Could you check a few things on this model? Use its own coordinates, in mm. A direction names the side the tool comes from. Coordinates: 2 decimals unless noted, no trailing zeros. Loops run counter-clockwise (first coordinate to the right, second up) from the corner with the lowest first, then second, coordinate; pieces in that order, holes last. Notation, with made-up numbers: (57, 41.5) -> (104, 41.5) arc R18 ccw to (104, 61.5) -> close; hole circle Ø5 at (63.5, 24). An arc over 180 degrees is marked (long way). One line per question, with ' | ' between items.
from build123d import *

# Parameters (mm, degrees)
SKETCH2_R           = 76.2
BOSS_EXTRUDE1_DEPTH = 50.8
CUT_EXTRUDE1_DEPTH  = 76.2
CUT_EXTRUDE2_DEPTH  = 76.2
SKETCH8_W           = 5.08
SKETCH8_H           = 5.08
CUT_EXTRUDE4_DEPTH  = 50.8
CUT_EXTRUDE5_DEPTH  = 51.8
SKETCH10_R          = 2.159
CUT_EXTRUDE6_DEPTH  = 25.4


with BuildPart() as part:
    # Sketch2 → Boss-Extrude1 (new body)
    with BuildSketch(Plane.XY):
        Circle(SKETCH2_R)
    extrude(amount=BOSS_EXTRUDE1_DEPTH)

    # Sketch4 → Cut-Extrude1 (cut)
    with BuildSketch(Plane.XY.offset(50.8)):
        with BuildLine():
            Line((-75.519629236, 10.16), (75.519629236, 10.16))
            ThreePointArc((75.519629236, 10.16), (0, 76.2), (-75.519629236, 10.16))
        make_face()
    extrude(amount=-CUT_EXTRUDE1_DEPTH, mode=Mode.SUBTRACT)

    # Sketch5 → Cut-Extrude2 (cut)
    with BuildSketch(Plane.XY.offset(50.8)):
        with BuildLine():
            Line((49.396930897, 5.08), (-49.396930897, 5.08))
            Line((-49.396930897, 5.08), (-49.396930897, -51.166371944))
            ThreePointArc((-49.396930897, -51.166371944), (-41.049983197, -58.077132157), (-31.75, -63.639546667))
            Line((-31.75, -63.639546667), (31.75, -63.639546667))
            ThreePointArc((31.75, -63.639546667), (41.049983197, -58.077132157), (49.396930897, -51.166371944))
            Line((49.396930897, -51.166371944), (49.396930897, 5.08))
        make_face()
    extrude(amount=-CUT_EXTRUDE2_DEPTH, mode=Mode.SUBTRACT)

    # Sketch8 → Cut-Extrude4 (cut)
    with BuildSketch(Plane.XY.offset(50.8)):
        with Locations((0, -66.179546667)):
            Rectangle(SKETCH8_W, SKETCH8_H)
    extrude(amount=-CUT_EXTRUDE4_DEPTH, mode=Mode.SUBTRACT)

    # Sketch9 → Cut-Extrude5 (cut, through all)
    with BuildSketch(Plane.XY.offset(50.8)):
        with BuildLine():
            Line((54.476930897, 5.08), (76.030478099, 5.08))
            ThreePointArc((76.030478099, 5.08), (71.480790805, -26.399555791), (54.476930897, -53.279489487))
            Line((54.476930897, -53.279489487), (54.476930897, 5.08))
        make_face()
        with BuildLine():
            Line((-54.476930897, 5.08), (-54.476930897, -53.279489487))
            ThreePointArc((-54.476930897, -53.279489487), (-71.480790805, -26.399555791), (-76.030478099, 5.08))
            Line((-76.030478099, 5.08), (-54.476930897, 5.08))
        make_face()
    extrude(amount=-CUT_EXTRUDE5_DEPTH, mode=Mode.SUBTRACT)

    # Sketch10 → Cut-Extrude6 (cut)
    with BuildSketch(Plane(origin=(0, 10.16, 0), x_dir=(1, 0, 0), z_dir=(0, 1, 0))):
        with Locations((-62.819629236, -12.7)):
            Circle(SKETCH10_R)
        with Locations((-62.819629236, -38.1)):
            Circle(SKETCH10_R)
        with Locations((62.819629236, -12.7)):
            Circle(SKETCH10_R)
        with Locations((62.819629236, -38.1)):
            Circle(SKETCH10_R)
    extrude(amount=-CUT_EXTRUDE6_DEPTH, mode=Mode.SUBTRACT)


solid = part.part
1) If we section it at C-C on z = 48: Please give me the cut outline in (x, y).
Data:
outline: (-76.03, 5.08) -> (-54.48, 5.08) -> (-54.48, -53.28) arc R76.2 ccw to (54.48, -53.28) -> (54.48, 5.08) -> (76.03, 5.08) arc R76.2 ccw to (75.52, 10.16) -> (-75.52, 10.16) arc R76.2 ccw to start; hole (-49.4, -51.17) arc R71.12 ccw to (-31.75, -63.64) -> (-2.54, -63.64) -> (-2.54, -68.72) -> (2.54, -68.72) -> (2.54, -63.64) -> (31.75, -63.64) arc R71.12 ccw to (49.4, -51.17) -> (49.4, 5.08) -> (-49.4, 5.08) -> close
2) If we section it at D-D on x = 38: Please give me the cut outline in (y, z).
Data:
outline: (-66.05, 0) -> (-60.12, 0) -> (-60.12, 50.8) -> (-66.05, 50.8) -> close; (5.08, 0) -> (10.16, 0) -> (10.16, 50.8) -> (5.08, 50.8) -> close
3) We'd pull the mould along Z, two halves only. Please class faces 1 (the face through (64.88, 7.66, 37.45)), 2 (the face through (-0.85, -76.195, 25.044)), 3 (the face through (0, 6, 50.8)): pulls with the +Z half, pulls with the -Z half, needs draft (parallel to the pull), parting line crosses it, or undercut.
Data:
face 1: undercut | face 2: needs draft | face 3: pulls with the +Z half
4) If we section it at B-B on y = -33.5: Please give me the cut outline in (x, z).
Data:
outline: (-54.48, 0) -> (-49.4, 0) -> (-49.4, 50.8) -> (-54.48, 50.8) -> close; (49.4, 0) -> (54.48, 0) -> (54.48, 50.8) -> (49.4, 50.8) -> close
5) If we section it at A-A on z = 38.1: Please give me the cut outline in (x, y).
Data:
outline: (-76.03, 5.08) -> (-64.98, 5.08) -> (-64.98, 10.16) -> (-75.52, 10.16) arc R76.2 ccw to start; (-60.66, 5.08) -> (-54.48, 5.08) -> (-54.48, -53.28) arc R76.2 ccw to (54.48, -53.28) -> (54.48, 5.08) -> (60.66, 5.08) -> (60.66, 10.16) -> (-60.66, 10.16) -> close; (64.98, 5.08) -> (76.03, 5.08) arc R76.2 ccw to (75.52, 10.16) -> (64.98, 10.16) -> close; hole (-49.4, -51.17) arc R71.12 ccw to (-31.75, -63.64) -> (-2.54, -63.64) -> (-2.54, -68.72) -> (2.54, -68.72) -> (2.54, -63.64) -> (31.75, -63.64) arc R71.12 ccw to (49.4, -51.17) -> (49.4, 5.08) -> (-49.4, 5.08) -> close
6) On a 3-axis mill with a long thin cutter (end or side, diameter ignored), from which of +Z, -Z, +X, -X, +Y, -Y can I reach the whole of each face in a straight line? I mean faces 4 (the face through (-54.477, -24, 26)), 5 (the face through (-64.977, 7.656, 38.005)), 6 (the face through (-41.17, -57.99, 25.76)), 7 (the face through (65, 5.08, 26)). Say none if no direction works.
Data:
face 4: +Z, -Z, -X, -Y | face 5: +Y, -Y | face 6: +Z, -Z | face 7: +Z, -Z, +X, -Y
7) I need wall thicknesses on line 1 along X through (y, z) = (-32.5, 12.5); line 2 along X through (y, z) = (8.35, 38.1); line 3 along X through (y, z) = (6, 38). Which ranges of each line are inside material? Lowest first, please. Write a range as from..to.
Data:
line 1: -54.48..-49.4, 49.4..54.48 | line 2: -75.74..-64.98, -60.66..60.66, 64.98..75.74 | line 3: -75.96..-64.98, -60.66..60.66, 64.98..75.96
8) I'm going to push flat-ended pins straight in: pin 1 Ø8 at (y, z) = (-29.5, 35.5) entering from +X; pin 2 Ø12 at (x, z) = (10.5, 36.5) entering from -Y; pin 3 Ø6 at (y, z) = (-33, 15) entering from -X; pin 4 Ø2.5 at (x, z) = (62.82, 12.7) entering from +Y. Where does each tip first touch, or does it pass through?
Data:
pin 1: x = 54.48 | pin 2: y = -76.07 | pin 3: x = -54.48 | pin 4: through
